The listing builds one solid part. Answer for the finished solid, in the listing's coordinates (mm). Face numbers are marked on the shaded views. Round coordinates to 2 decimals unless told otherwise and drop trailing zeros. Order: outer loops, then holes, each group sorted by start corner. A loop starts at its lowest first (then second) coordinate and runs counter-clockwise, first axis right, second up. Notation, with made-up numbers: (86, -34) - (125, -34) arc R20 ccw to (125, -8) - close; hole circle Ø8 at (43.5, 35.5). An arc over 180 degrees is marked (long way). One line per item, written item: value. Start each with the question number.
1. Flat-ended cylindrical pins translate along their axes: P1, Ø2, axis at y = 16, z = -132, coming from the -X side; P2, Ø1.5, axis at x = 141.5, y = 18, coming from the -Z side; P3, Ø1.6, axis at y = 16, z = -18, coming from the +X side. Find the tip coordinate at first contact, or state that the pin passes through.
2. For a pull along Z with two mould halves and no side action, classify the marked faces 1, 2 and 3 as released by +Z, released by -Z, zero draft, split by the parting line, or undercut.
3. Straight lines are drawn through the part: line 1 (Z direction, x = 317, y = 17.9); line 2 (Z direction, x = 280, y = 15.5); line 3 (X direction, y = 11.25, z = -110). For each, find the intervals that lie inside material, in ascending order.
4. Section A-A, the plane x = 63 is taken. Give the vertices of the cut face in (y, z), then the cut area to 3 significant figures.
5. Section B-B, the plane x = 253 is taken. Give the vertices of the cut face in (y, z), then the cut area to 4 significant figures.
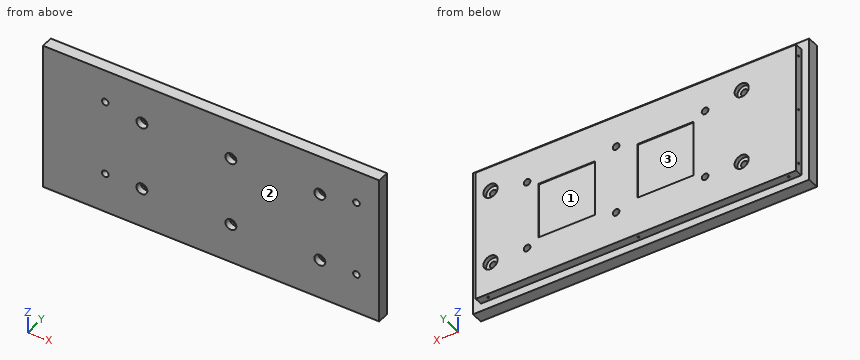
from build123d import *

# Parameters (mm, degrees)
SKETCH1_W                                            = 340
SKETCH1_H                                            = 150
BOSS_EXTRUDE1_DEPTH                                  = 20
LASERCAVITYMOUNTINGHOLE_CBORE_FOR_1_4_SO_D           = 6.7564
LASERCAVITYMOUNTINGHOLE_CBORE_FOR_1_4_SO_CBORE_D     = 11.1125
LASERCAVITYMOUNTINGHOLE_CBORE_FOR_1_4_SO_CBORE_DEPTH = 6.35
SKETCH5_W                                            = 57
SKETCH5_H                                            = 57
TEC_GROOVE_DEPTH                                     = 1
SKETCH6_W                                            = 340
SKETCH6_H                                            = 8
WALL1_DEPTH                                          = 8
SKETCH7_W                                            = 142
SKETCH7_H                                            = 8
WALL2_DEPTH                                          = 8
SKETCH9_W                                            = 332
SKETCH9_H                                            = 8
WALL3_DEPTH                                          = 8
SKETCH10_W                                           = 134
SKETCH10_H                                           = 8
WALL4_DEPTH                                          = 8
F_2_56_TAPPED_HOLE1_D                                = 1.778
F_2_56_TAPPED_HOLE1_DEPTH                            = 15
F_2_56_TAPPED_HOLE1_TIP                              = 0.53416509
F_2_56_TAPPED_HOLE2_D                                = 1.778
F_2_56_TAPPED_HOLE2_DEPTH                            = 15
F_2_56_TAPPED_HOLE2_TIP                              = 0.53416509
F_2_56_TAPPED_HOLE3_D                                = 1.778
F_2_56_TAPPED_HOLE3_DEPTH                            = 15
F_2_56_TAPPED_HOLE3_TIP                              = 0.53416509
F_2_56_TAPPED_HOLE4_D                                = 1.778
F_2_56_TAPPED_HOLE4_DEPTH                            = 15
F_2_56_TAPPED_HOLE4_TIP                              = 0.53416509
OPTICALTABLEMOUNTINGHOLES_CBORE_FOR_1_4_D            = 6.7564
OPTICALTABLEMOUNTINGHOLES_CBORE_FOR_1_4_DEPTH        = 20
OPTICALTABLEMOUNTINGHOLES_CBORE_FOR_1_4_CBORE_D      = 14.2875
OPTICALTABLEMOUNTINGHOLES_CBORE_FOR_1_4_CBORE_DEPTH  = 4.191
OPTICALTABLEMOUNTINGHOLES_CBORE_FOR_1_4_TIP          = 2.029827343


with BuildPart() as part:
    # Sketch1 → Boss-Extrude1 (new body)
    with BuildSketch(Plane(origin=(0, 0, 0), x_dir=(1, 0, 0), z_dir=(0, 1, 0))):
        with Locations((170, 75)):
            Rectangle(SKETCH1_W, SKETCH1_H)
    extrude(amount=BOSS_EXTRUDE1_DEPTH)

    # LaserCavityMountingHole_CBORE for 1/4 Socket Head Cap Screw1 (through all)
    with Locations(Plane(origin=(0, 0, 0), x_dir=(-1, 0, 0), z_dir=(0, -1, 0))):
        with Locations((-100, 40), (-190, 40), (-280, 40), (-280, 110), (-190, 110), (-100, 110)):
            CounterBoreHole(LASERCAVITYMOUNTINGHOLE_CBORE_FOR_1_4_SO_D / 2, LASERCAVITYMOUNTINGHOLE_CBORE_FOR_1_4_SO_CBORE_D / 2, LASERCAVITYMOUNTINGHOLE_CBORE_FOR_1_4_SO_CBORE_DEPTH)

    # Sketch5 → TEC_groove (cut)
    with BuildSketch(Plane(origin=(0, 20, 0), x_dir=(1, 0, 0), z_dir=(0, 1, 0))):
        with Locations((140, 75)):
            Rectangle(SKETCH5_W, SKETCH5_H)
        with Locations((240, 75)):
            Rectangle(SKETCH5_W, SKETCH5_H)
    extrude(amount=-TEC_GROOVE_DEPTH, mode=Mode.SUBTRACT)

    # Sketch6 → Wall1 (cut)
    with BuildSketch(Plane.XY):
        with Locations((170, 16)):
            Rectangle(SKETCH6_W, SKETCH6_H)
    extrude(amount=-WALL1_DEPTH, mode=Mode.SUBTRACT)

    # Sketch7 → Wall2 (cut)
    with BuildSketch(Plane(origin=(340, 0, 0), x_dir=(0, 0, -1), z_dir=(1, 0, 0))):
        with Locations((79, 16)):
            Rectangle(SKETCH7_W, SKETCH7_H)
    extrude(amount=-WALL2_DEPTH, mode=Mode.SUBTRACT)

    # Sketch9 → Wall3 (cut)
    with BuildSketch(Plane(origin=(0, 0, -150), x_dir=(-1, 0, 0), z_dir=(0, 0, -1))):
        with Locations((-166, 16)):
            Rectangle(SKETCH9_W, SKETCH9_H)
    extrude(amount=-WALL3_DEPTH, mode=Mode.SUBTRACT)

    # Sketch10 → Wall4 (cut)
    with BuildSketch(Plane.ZY):
        with Locations((-75, 16)):
            Rectangle(SKETCH10_W, SKETCH10_H)
    extrude(amount=-WALL4_DEPTH, mode=Mode.SUBTRACT)

    # #2-56 Tapped Hole1
    with Locations(Plane.XY.offset(-8)):
        with Locations((18, 16), (322, 16), (170, 16)):
            Hole(F_2_56_TAPPED_HOLE1_D / 2, depth=F_2_56_TAPPED_HOLE1_DEPTH)
            with Locations((0, 0, -(F_2_56_TAPPED_HOLE1_DEPTH + F_2_56_TAPPED_HOLE1_TIP / 2))):  # 118° drill point
                Cone(0, F_2_56_TAPPED_HOLE1_D / 2, F_2_56_TAPPED_HOLE1_TIP, mode=Mode.SUBTRACT)

    # #2-56 Tapped Hole2
    with Locations(Plane(origin=(8, 16, -132), x_dir=(0, 0, -1), z_dir=(-1, 0, 0))):
        with Locations((0, 0), (-114, 0), (-57, 0)):
            Hole(F_2_56_TAPPED_HOLE2_D / 2, depth=F_2_56_TAPPED_HOLE2_DEPTH)
            with Locations((0, 0, -(F_2_56_TAPPED_HOLE2_DEPTH + F_2_56_TAPPED_HOLE2_TIP / 2))):  # 118° drill point
                Cone(0, F_2_56_TAPPED_HOLE2_D / 2, F_2_56_TAPPED_HOLE2_TIP, mode=Mode.SUBTRACT)

    # #2-56 Tapped Hole3
    with Locations(Plane(origin=(0, 0, -142), x_dir=(-1, 0, 0), z_dir=(0, 0, -1))):
        with Locations((-322, 16), (-18, 16), (-170, 16)):
            Hole(F_2_56_TAPPED_HOLE3_D / 2, depth=F_2_56_TAPPED_HOLE3_DEPTH)
            with Locations((0, 0, -(F_2_56_TAPPED_HOLE3_DEPTH + F_2_56_TAPPED_HOLE3_TIP / 2))):  # 118° drill point
                Cone(0, F_2_56_TAPPED_HOLE3_D / 2, F_2_56_TAPPED_HOLE3_TIP, mode=Mode.SUBTRACT)

    # #2-56 Tapped Hole4
    with Locations(Plane(origin=(332, 0, 0), x_dir=(0, 0, -1), z_dir=(1, 0, 0))):
        with Locations((18, 16), (132, 16), (75, 16)):
            Hole(F_2_56_TAPPED_HOLE4_D / 2, depth=F_2_56_TAPPED_HOLE4_DEPTH)
            with Locations((0, 0, -(F_2_56_TAPPED_HOLE4_DEPTH + F_2_56_TAPPED_HOLE4_TIP / 2))):  # 118° drill point
                Cone(0, F_2_56_TAPPED_HOLE4_D / 2, F_2_56_TAPPED_HOLE4_TIP, mode=Mode.SUBTRACT)

    # OpticalTableMountingHoles_CBORE for 1/4 Binding Head Machine Screw1
    with Locations(Plane(origin=(0, 20, 0), x_dir=(1, 0, 0), z_dir=(0, 1, 0))):
        with Locations((63, 109.6), (317, 109.6), (317, 33.4), (63, 33.4)):
            CounterBoreHole(OPTICALTABLEMOUNTINGHOLES_CBORE_FOR_1_4_D / 2, OPTICALTABLEMOUNTINGHOLES_CBORE_FOR_1_4_CBORE_D / 2, OPTICALTABLEMOUNTINGHOLES_CBORE_FOR_1_4_CBORE_DEPTH, depth=OPTICALTABLEMOUNTINGHOLES_CBORE_FOR_1_4_DEPTH)
            with Locations((0, 0, -(OPTICALTABLEMOUNTINGHOLES_CBORE_FOR_1_4_DEPTH + OPTICALTABLEMOUNTINGHOLES_CBORE_FOR_1_4_TIP / 2))):  # 118° drill point
                Cone(0, OPTICALTABLEMOUNTINGHOLES_CBORE_FOR_1_4_D / 2, OPTICALTABLEMOUNTINGHOLES_CBORE_FOR_1_4_TIP, mode=Mode.SUBTRACT)


solid = part.part
Answer list:
1. P1: stops at x = 8
1. P2: stops at z = -142
1. P3: stops at x = 316.95
2. face 1: undercut
2. face 2: zero draft
2. face 3: undercut
3. line 1: z = -142 to -116.74, -102.46 to -40.54, -26.26 to -8
3. line 2: z = -142 to -113.38, -106.62 to -43.38, -36.62 to -8
3. line 3: x = 0 to 59.65, 66.35 to 96.62, 103.38 to 186.62, 193.38 to 276.62, 283.38 to 313.65, 320.35 to 340
4. outline: (0, -150) - (12, -150) - (12, -142) - (20, -142) - (20, -116.74) - (15.81, -116.74) - (15.81, -112.98) - (0, -112.98) - close; (0, -106.22) - (15.81, -106.22) - (15.81, -102.46) - (20, -102.46) - (20, -40.54) - (15.81, -40.54) - (15.81, -36.78) - (0, -36.78) - close; (0, -30.02) - (15.81, -30.02) - (15.81, -26.26) - (20, -26.26) - (20, -8) - (12, -8) - (12, 0) - (0, 0) - close
4. area: 2,540 mm²
5. outline: (0, -150) - (12, -150) - (12, -142) - (20, -142) - (20, -103.5) - (19, -103.5) - (19, -46.5) - (20, -46.5) - (20, -8) - (12, -8) - (12, 0) - (0, 0) - close
5. area: 2,815 mm²
